Can you work these out from the model? Positions are in its coordinate system, mm. Face numbers are marked on the shaded views. A direction names the side the tool comes from. Give positions to 0.01 mm unless a question says otherwise; leave off trailing zeros. Order: outer loops, then holes, each group sorted by start corner. A loop starts at its lowest first (then second) coordinate and runs counter-clockwise, first axis right, second up. Notation, with made-up numbers: M -15,54 L -5,54 A25 cw -5,73 Z; hole C 19.25,2.25 d3. An arc over 180 degrees is marked long. Write each question's results on one line, items separated by ' | '.
from build123d import *

# Parameters (mm, degrees)
F0_W      = 51
F0_H      = 56
F1_DEPTH  = 30
F2_T      = -2
F3_R      = 5
F4_W      = 26.5
F4_H      = 16
F5_DEPTH  = 2.001
F6_SIZE   = 0.5
F7_W      = 42.5
F7_H      = 2
F8_DEPTH  = 26
F9_R      = 0.5
F10_W     = 9
F10_H     = 3
F11_DEPTH = 3
F12_W     = 2
F12_H     = 20
F13_DEPTH = 5
F12_W_2   = 1.5
F14_DEPTH = 7
F15_W     = 3
F15_H     = 8
F16_DEPTH = 6.54
F17_R     = 2.25
F18_DEPTH = 2.001
F15_W_2   = 1.5
F19_DEPTH = 7.54
F20_R     = 0.5
F21_DEPTH = 5
F22_R     = 1.15
F23_DEPTH = 2.5
F24_R     = 0.75
F25_DEPTH = 28
F26_W     = 2
F26_H     = 4.6
F27_DEPTH = 2


with BuildPart() as f1:
    # F0 (on Front) → F1 (new body)
    with BuildSketch(Plane.XZ):
        with Locations((25.5, 28)):
            Rectangle(F0_W, F0_H)
    extrude(amount=F1_DEPTH)

    # F2
    f2_openings = [f1.faces().sort_by_distance(p)[0] for p in [
        (25.5, -30, 28),
    ]]
    offset(amount=F2_T, openings=f2_openings)

    # F3
    f3_edges = [f1.edges().sort_by_distance(p)[0] for p in [
        (0, -15, 56),
        (0, -15, 0),
        (51, -15, 0),
        (51, -15, 56),
    ]]
    fillet(f3_edges, radius=F3_R)

    # F4 (on face) → F5 (cut, through all)
    with BuildSketch(Plane.XZ.offset(2)):
        with Locations((25.5, 39.58)):
            Rectangle(F4_W, F4_H)
    extrude(amount=-F5_DEPTH, mode=Mode.SUBTRACT)

    # F6
    f6_edges = [f1.edges().sort_by_distance(p)[0] for p in [
        (25.5, 0, 47.58),
        (38.75, 0, 39.58),
        (25.5, 0, 31.58),
        (12.25, 0, 39.58),
    ]]
    chamfer(f6_edges, length=F6_SIZE)

    # F7 (on face) → F8 (join)
    with BuildSketch(Plane.XZ.offset(2)):
        with Locations((23.25, 12)):
            Rectangle(F7_W, F7_H)
    extrude(amount=F8_DEPTH)

    # F9
    f9_edges = [f1.edges().sort_by_distance(p)[0] for p in [
        (44.5, -15, 11),
        (44.5, -15, 13),
    ]]
    fillet(f9_edges, radius=F9_R)

    # F10 (on face) → F11 (cut)
    with BuildSketch(Plane(origin=(0, 0, 0), x_dir=(0, -1, 0), z_dir=(-1, 0, 0))):
        with Locations((18.4, 16)):
            Rectangle(F10_W, F10_H)
    extrude(amount=-F11_DEPTH, mode=Mode.SUBTRACT)

    # F12 (on face) → F13 (join)
    with BuildSketch(Plane.XZ.offset(2)):
        with Locations((9.65, 39.58)):
            Rectangle(F12_W, F12_H)
        with Locations((41.35, 39.58)):
            Rectangle(F12_W, F12_H)
    extrude(amount=F13_DEPTH)

    # F12 (on face) → F14 (join)
    with BuildSketch(Plane.XZ.offset(2)):
        with Locations((7.9, 39.58)):
            Rectangle(F12_W_2, F12_H)
        with Locations((43.1, 39.58)):
            Rectangle(F12_W_2, F12_H)
    extrude(amount=F14_DEPTH)

    # F15 (on face) → F16 (join)
    with BuildSketch(Plane.XZ.offset(2)):
        with Locations((10, 20)):
            Rectangle(F15_W, F15_H)
        with Locations((41, 20)):
            Rectangle(F15_W, F15_H)
    extrude(amount=F16_DEPTH)

    # F17 (on face) → F18 (cut, through all)
    with BuildSketch(Plane.XZ.offset(2)):
        with Locations((15.4, 20)):
            Circle(F17_R)
        with Locations((25.5, 20)):
            Circle(F17_R)
        with Locations((35.6, 20)):
            Circle(F17_R)
    extrude(amount=-F18_DEPTH, mode=Mode.SUBTRACT)

    # F15 (on face) → F19 (join)
    with BuildSketch(Plane.XZ.offset(2)):
        with Locations((7.75, 20)):
            Rectangle(F15_W_2, F15_H)
        with Locations((43.25, 20)):
            Rectangle(F15_W_2, F15_H)
    extrude(amount=F19_DEPTH)

    # F20 (on face) → F21 (cut)
    with BuildSketch(Plane.XZ.offset(8.54)):
        with Locations((10.551, 20)):
            Circle(F20_R)
        with Locations((40.449, 20)):
            Circle(F20_R)
    extrude(amount=-F21_DEPTH, mode=Mode.SUBTRACT)

    # F22 (on face) → F23 (join)
    with BuildSketch(Plane.XZ.offset(2)):
        with Locations((15.2, 49.51)):
            Circle(F22_R)
        with Locations((35.8, 49.51)):
            Circle(F22_R)
        with Locations((35.8, 26.01)):
            Circle(F22_R)
        with Locations((15.2, 26.01)):
            Circle(F22_R)
    extrude(amount=F23_DEPTH)

    # F24 (on face) → F25 (join)
    with BuildSketch(Plane.XZ.offset(2)):
        with BuildLine():
            Line((5.5, 54), (2, 54))
            Line((2, 54), (2, 50.5))
            ThreePointArc((2, 50.5), (4.474874, 51.525126), (5.5, 54))
        make_face()
        with Locations((3.25, 52.75)):
            Circle(F24_R, mode=Mode.SUBTRACT)
        with BuildLine():
            Line((49, 50.5), (49, 54))
            Line((49, 54), (45.5, 54))
            ThreePointArc((45.5, 54), (46.525126, 51.525126), (49, 50.5))
        make_face()
        with Locations((47.75, 52.75)):
            Circle(F24_R, mode=Mode.SUBTRACT)
        with BuildLine():
            Line((45.5, 2), (49, 2))
            Line((49, 2), (49, 5.5))
            ThreePointArc((49, 5.5), (46.525126, 4.474874), (45.5, 2))
        make_face()
        with Locations((47.75, 3.25)):
            Circle(F24_R, mode=Mode.SUBTRACT)
        with BuildLine():
            Line((2, 5.5), (2, 2))
            Line((2, 2), (5.5, 2))
            ThreePointArc((5.5, 2), (4.474874, 4.474874), (2, 5.5))
        make_face()
        with Locations((3.25, 3.25)):
            Circle(F24_R, mode=Mode.SUBTRACT)
    extrude(amount=F25_DEPTH)

    # F26 (on face) → F27 (cut)
    with BuildSketch(Plane.YZ.offset(51)):
        with Locations((-20, 22.3)):
            Rectangle(F26_W, F26_H)
    extrude(amount=-F27_DEPTH, mode=Mode.SUBTRACT)


solid = f1.part
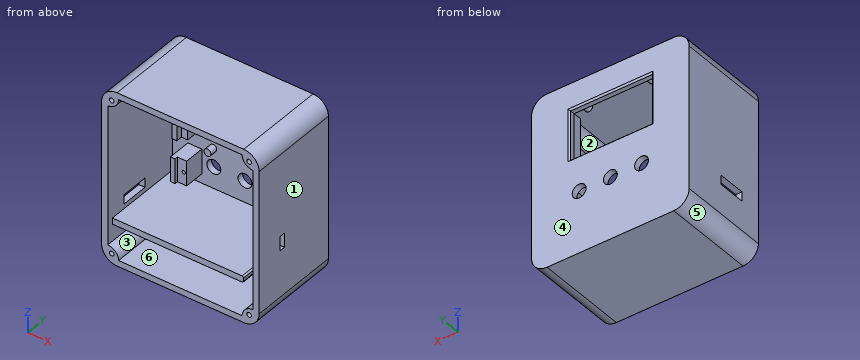
(1) Imagine slicing it at A-A, the plane x = 25.5. Write out the boundary of the cut face in (y, z).
Data:
outline: M -30,0 L 0,0 L 0,17.75 L -2,17.75 L -2,13 L -28,13 L -28,11 L -2,11 L -2,2 L -30,2 Z; M -30,54 L -2,54 L -2,47.58 L -0.5,47.58 L 0,48.08 L 0,56 L -30,56 Z; M -2,22.25 L 0,22.25 L 0,31.08 L -0.5,31.58 L -2,31.58 Z
(2) We'd pull the mould along Z, two halves only. Please class the marked faces 3, 4, 5 and 6: +Z half, -Z half, draft (parallel to the pull), parting line (faces both ways), or undercut.
Data:
face 3: undercut | face 4: draft | face 5: -Z half | face 6: undercut
(3) Imagine slicing it at B-B, the plane z = 44. Write out the boundary of the cut face in (x, y), plus the area to 3 significant figures.
Data:
outline: M 0,-30 L 2,-30 L 2,-2 L 7.15,-2 L 7.15,-9 L 8.65,-9 L 8.65,-7 L 10.65,-7 L 10.65,-2 L 12.25,-2 L 12.25,-0.5 L 11.75,0 L 0,0 Z; M 38.75,-2 L 40.35,-2 L 40.35,-7 L 42.35,-7 L 42.35,-9 L 43.85,-9 L 43.85,-2 L 49,-2 L 49,-30 L 51,-30 L 51,0 L 39.25,0 L 38.75,-0.5 Z | area: 202 mm2
(4) I need wall thicknesses on L1, parallel to Z at x = 22.5, y = -19; L2, parallel to Z at x = 43, y = -2.25; L3, parallel to X at y = -4, z = 25. Which ranges of each line are inside material? Lowest first, please. Write a range as from..to.
Data:
L1: z = 0..2, 11..13, 54..56 | L2: z = 0..2, 11..13, 16..24, 29.58..49.58, 54..56 | L3: x = 0..2, 14.65..15.75, 35.25..36.35, 49..51
(5) Imagine slicing it at D-D, the plane z = 26.01. Write out the boundary of the cut face in (x, y), plus the area to 4 significant figures.
Data:
outline: M 0,-30 L 2,-30 L 2,-2 L 14.05,-2 L 14.05,-4.5 L 16.35,-4.5 L 16.35,-2 L 34.65,-2 L 34.65,-4.5 L 36.95,-4.5 L 36.95,-2 L 49,-2 L 49,-30 L 51,-30 L 51,0 L 0,0 Z | area: 225.5 mm2
(6) Will these pins go through, and if not, where does the flat tip stop? P1, Ø1.6, axis at x = 43, z = 40, coming from the -Y side; P2, Ø14, axis at x = 22, z = 36.5, coming from the -Y side; P3, Ø1.6, axis at x = 10, z = 35.5, coming from the -Y side.
Data:
P1: stops at y = -9 | P2: stops at y = -2 | P3: stops at y = -7
(7) Imagine slicing it at C-C, the plane y = -26. Write out the boundary of the cut face in (x, z).
Data:
outline: M 0,5 A5 ccw 5,0 L 46,0 A5 ccw 51,5 L 51,51 A5 ccw 46,56 L 5,56 A5 ccw 0,51 Z; hole M 2,5.5 A3.5 cw 5.5,2 L 45.5,2 A3.5 cw 49,5.5 L 49,50.5 A3.5 cw 45.5,54 L 5.5,54 A3.5 cw 2,50.5 L 2,13 L 44,13 A0.5 cw 44.5,12.5 L 44.5,11.5 A0.5 cw 44,11 L 2,11 Z; hole C 3.25,3.25 d1.5; hole C 3.25,52.75 d1.5; hole C 47.75,3.25 d1.5; hole C 47.75,52.75 d1.5
(8) For the marked faces 1 and 2, which set-ups out of +Z, -Z, +X, -X, +Y, -Y let a thin tool reach every point of the face, with its end or its side?
Data:
face 1: +Z, -Z, +X, +Y, -Y | face 2: -Y
